```python
from build123d import *

# Parameters (mm, degrees)
SKETCH1_W                 = 64
SKETCH1_H                 = 10
SKETCH1_R                 = 1.8
SKETCH1_R_2               = 2.625
BOSS_EXTRUDE1_DEPTH       = 4
BOSS_EXTRUDE2_START       = 4
BOSS_EXTRUDE2_OUTLINE_R   = 3.5
BOSS_EXTRUDE2_OUTLINE_R_2 = 2.625
BOSS_EXTRUDE2_DEPTH       = 0.5


# Read off the part's stored shape, not the designer's step: Boss-Extrude2
with BuildPart() as part:
    # Sketch1 → Boss-Extrude1 (new body)
    with BuildSketch(Plane(origin=(0, 0, 0), x_dir=(1, 0, 0), z_dir=(0, 1, 0))):
        with Locations((32, 5)):
            Rectangle(SKETCH1_W, SKETCH1_H)
        with Locations(Location((3, 5, 0), (0, 0, 270))):
            Circle(SKETCH1_R, mode=Mode.SUBTRACT)
        with Locations(Location((16, 5, 0), (0, 0, 270))):
            Circle(SKETCH1_R_2, mode=Mode.SUBTRACT)
        with Locations(Location((61, 5, 0), (0, 0, 90))):
            Circle(SKETCH1_R, mode=Mode.SUBTRACT)
        with Locations(Location((48, 5, 0), (0, 0, 90))):
            Circle(SKETCH1_R_2, mode=Mode.SUBTRACT)
    extrude(amount=BOSS_EXTRUDE1_DEPTH)

    # Boss-Extrude2 outline → Boss-Extrude2 (add)
    # profile 1 of 2: a face of its own
    with BuildSketch(Plane(origin=(0, 0, 0), x_dir=(1, 0, 0), z_dir=(0, 1, 0)).offset(BOSS_EXTRUDE2_START)):
        with Locations((16, 5)):
            Circle(BOSS_EXTRUDE2_OUTLINE_R)
        with Locations((16, 5)):
            Circle(BOSS_EXTRUDE2_OUTLINE_R_2, mode=Mode.SUBTRACT)
    # profile 2 of 2: a face of its own
    with BuildSketch(Plane(origin=(0, 0, 0), x_dir=(1, 0, 0), z_dir=(0, 1, 0)).offset(BOSS_EXTRUDE2_START)):
        with Locations((48, 5)):
            Circle(BOSS_EXTRUDE2_OUTLINE_R)
        with Locations((48, 5)):
            Circle(BOSS_EXTRUDE2_OUTLINE_R_2, mode=Mode.SUBTRACT)
    extrude(amount=BOSS_EXTRUDE2_DEPTH)


solid = part.part
```
Here's how the part is built. I have some questions about the finished solid (model axes, mm). A direction names the side the tool comes from. Coordinates: 2 decimals unless noted, no trailing zeros. Order: outer loops, then holes, each group sorted by start corner. A loop starts at its lowest first (then second) coordinate and runs counter-clockwise, first axis right, second up. Notation, with made-up numbers: M -7,12 L 40,12 A10 ccw 40,21 Z; hole C -18.5,39 d6. An arc over 180 degrees is marked long. Answer as a JSON object with one key per item and string values. Group by question number.
(1) Which directions (+Z, -Z, +X, -X, +Y, -Y) give clear straight access to the entire face, cutting with the end or side of a thin tool? Please do faces 1 (the face through (19.233, 4.246, -3.659)), 2 (the face through (32, 2, 0)).
(2) Suppose I cut it at B-B, the plane y = 2.8. Please give me the cut outline in (x, z) (3 decimals).
(3) Suppose I cut it at C-C, the plane x = 22. Please give me the cut outline in (y, z).
(4) I need wall thicknesses on probe 1 along X at (y, z) = (1.35, -5) (3 decimals); probe 2 along Z at (x, y) = (61, 3.1); probe 3 along X at (y, z) = (2.8, -3). Which ranges of each line are inside material? Lowest first, please.
(5) If we mould it in two halves opening along X, with no side actions, what happens to faces 3 (the face through (17, 4.5, -8)), 4 (the face through (44.503, 4.246, -5.154)), 5 (the face through (64, 2, -5))? For each: released by +X, released by -X, zero draft, split by the parting line, or undercut.
(6) Suppose I cut it at A-A, the plane x = 61. Please give me the cut outline in (y, z).
(7) For pin 1 (2 mm diameter, centred on x = 25, z = -6, fed in from -Y); pin 2 (6 mm diameter, centred on x = 35, z = -8, fed in from +Y), each with a flat end and sliding along its axis, tell me the tip position at first contact or that it passes through.
Values found:
{
 "1": {"face 1": "+Y", "face 2": "+Z, +X, -X, +Y, -Y"},
 "2": {"outline": "M 0,-10 L 64,-10 L 64,0 L 0,0 Z; hole C 3,-5 d3.6; hole C 16,-5 d5.25; hole C 48,-5 d5.25; hole C 61,-5 d3.6"},
 "3": {"outline": "M 0,-10 L 4,-10 L 4,0 L 0,0 Z"},
 "4": {"probe 1": "x = 0 to 1.2, 4.8 to 13.375, 18.625 to 45.375, 50.625 to 59.2, 62.8 to 64", "probe 2": "z = -10 to -6.8, -3.2 to 0", "probe 3": "x = 0 to 14.3, 17.7 to 46.3, 49.7 to 64"},
 "5": {"face 3": "zero draft", "face 4": "undercut", "face 5": "released by +X"},
 "6": {"outline": "M 0,-10 L 4,-10 L 4,-6.8 L 0,-6.8 Z; M 0,-3.2 L 4,-3.2 L 4,0 L 0,0 Z"},
 "7": {"pin 1": "stops at y = 0", "pin 2": "stops at y = 4"}
}
